Check sheet for the modelled part. Datum: model origin and axes. Units: mm. Coordinates: 2 decimals unless noted, no trailing zeros. Loops run counter-clockwise (first coordinate to the right, second up) from the corner with the lowest first, then second, coordinate; pieces in that order, holes last. Notation, with made-up numbers: M -32.5,21.5 L 19.5,21.5 A16 ccw 19.5,27.5 Z; hole C 24.5,71 d2. An arc over 180 degrees is marked long. Return JSON: item names as keys, results as strings.
from build123d import *

# Parameters (mm, degrees)
ESQUISSE1_R             = 40
ESQUISSE1_R_2           = 5.5
BOSS_EXTRU_1_DEPTH      = 10
BOSS_EXTRU_2_START      = -7
ESQUISSE2_R             = 40
BOSS_EXTRU_2_DEPTH      = 7
ESQUISSE3_R             = 15
BOSS_EXTRU_3_DEPTH      = 20
CONG_1_R                = 10
ESQUISSE4_R             = 4.875
ENL_V_MAT_EXTRU_1_DEPTH = 16


with BuildPart() as part:
    # Esquisse1 → Boss.-Extru.1 (new body)
    with BuildSketch(Plane.YZ):
        with Locations(Location((0, 0, 0), (0, 0, 270))):
            Circle(ESQUISSE1_R)
        with Locations(Location((0, 32, 0), (0, 0, 270))):
            Circle(ESQUISSE1_R_2, mode=Mode.SUBTRACT)
        with Locations(Location((12.245869836, 29.56414504, 0), (0, 0, 270))):
            Circle(ESQUISSE1_R_2, mode=Mode.SUBTRACT)
        with Locations(Location((22.627416998, 22.627416998, 0), (0, 0, 270))):
            Circle(ESQUISSE1_R_2, mode=Mode.SUBTRACT)
        with Locations(Location((29.56414504, 12.245869836, 0), (0, 0, 270))):
            Circle(ESQUISSE1_R_2, mode=Mode.SUBTRACT)
        with Locations(Location((32, 0, 0), (0, 0, 270))):
            Circle(ESQUISSE1_R_2, mode=Mode.SUBTRACT)
        with Locations(Location((29.56414504, -12.245869836, 0), (0, 0, 270))):
            Circle(ESQUISSE1_R_2, mode=Mode.SUBTRACT)
        with Locations(Location((22.627416998, -22.627416998, 0), (0, 0, 270))):
            Circle(ESQUISSE1_R_2, mode=Mode.SUBTRACT)
        with Locations(Location((12.245869836, -29.56414504, 0), (0, 0, 270))):
            Circle(ESQUISSE1_R_2, mode=Mode.SUBTRACT)
        with Locations(Location((0, -32, 0), (0, 0, 270))):
            Circle(ESQUISSE1_R_2, mode=Mode.SUBTRACT)
        with Locations(Location((-12.245869836, -29.56414504, 0), (0, 0, 270))):
            Circle(ESQUISSE1_R_2, mode=Mode.SUBTRACT)
        with Locations(Location((-22.627416998, -22.627416998, 0), (0, 0, 270))):
            Circle(ESQUISSE1_R_2, mode=Mode.SUBTRACT)
        with Locations(Location((-29.56414504, -12.245869836, 0), (0, 0, 270))):
            Circle(ESQUISSE1_R_2, mode=Mode.SUBTRACT)
        with Locations(Location((-32, 0, 0), (0, 0, 270))):
            Circle(ESQUISSE1_R_2, mode=Mode.SUBTRACT)
        with Locations(Location((-29.56414504, 12.245869836, 0), (0, 0, 270))):
            Circle(ESQUISSE1_R_2, mode=Mode.SUBTRACT)
        with Locations(Location((-22.627416998, 22.627416998, 0), (0, 0, 270))):
            Circle(ESQUISSE1_R_2, mode=Mode.SUBTRACT)
        with Locations(Location((-12.245869836, 29.56414504, 0), (0, 0, 270))):
            Circle(ESQUISSE1_R_2, mode=Mode.SUBTRACT)
        with Locations(Location((-11.429260712, 17.105097445, 0), (0, 0, 270))):
            Circle(ESQUISSE1_R_2, mode=Mode.SUBTRACT)
        with Locations(Location((4.013422643, 20.17683815, 0), (0, 0, 270))):
            Circle(ESQUISSE1_R_2, mode=Mode.SUBTRACT)
        with Locations(Location((17.105097445, 11.429260712, 0), (0, 0, 270))):
            Circle(ESQUISSE1_R_2, mode=Mode.SUBTRACT)
        with Locations(Location((20.17683815, -4.013422643, 0), (0, 0, 270))):
            Circle(ESQUISSE1_R_2, mode=Mode.SUBTRACT)
        with Locations(Location((11.429260712, -17.105097445, 0), (0, 0, 270))):
            Circle(ESQUISSE1_R_2, mode=Mode.SUBTRACT)
        with Locations(Location((-4.013422643, -20.17683815, 0), (0, 0, 270))):
            Circle(ESQUISSE1_R_2, mode=Mode.SUBTRACT)
        with Locations(Location((-17.105097445, -11.429260712, 0), (0, 0, 270))):
            Circle(ESQUISSE1_R_2, mode=Mode.SUBTRACT)
        with Locations(Location((-20.17683815, 4.013422643, 0), (0, 0, 270))):
            Circle(ESQUISSE1_R_2, mode=Mode.SUBTRACT)
        with Locations(Location((5.527683242, 8.272762594, 0), (0, 0, 270))):
            Circle(ESQUISSE1_R_2, mode=Mode.SUBTRACT)
        with Locations(Location((8.272762594, -5.527683242, 0), (0, 0, 270))):
            Circle(ESQUISSE1_R_2, mode=Mode.SUBTRACT)
        with Locations(Location((-5.527683242, -8.272762594, 0), (0, 0, 270))):
            Circle(ESQUISSE1_R_2, mode=Mode.SUBTRACT)
        with Locations(Location((-8.272762594, 5.527683242, 0), (0, 0, 270))):
            Circle(ESQUISSE1_R_2, mode=Mode.SUBTRACT)
    extrude(amount=BOSS_EXTRU_1_DEPTH)

    # Esquisse2 → Boss.-Extru.2 (add)
    with BuildSketch(Plane.YZ.offset(10).offset(BOSS_EXTRU_2_START)):
        with Locations(Location((0, 0, 0), (0, 0, 270))):
            Circle(ESQUISSE2_R)
    extrude(amount=BOSS_EXTRU_2_DEPTH)

    # Esquisse3 → Boss.-Extru.3 (add)
    with BuildSketch(Plane.YZ.offset(10)):
        with Locations(Location((0, 0, 0), (0, 0, 270))):
            Circle(ESQUISSE3_R)
    extrude(amount=BOSS_EXTRU_3_DEPTH)

    # Congé1
    cong_1_edges = [part.edges().sort_by_distance(p)[0] for p in [
        (10, 0, 15),
    ]]
    fillet(cong_1_edges, radius=CONG_1_R)

    # Esquisse4 → Enlèv. mat.-Extru.1 (cut)
    with BuildSketch(Plane.YZ.offset(30)):
        with Locations(Location((0, 0, 0), (0, 0, 270))):
            Circle(ESQUISSE4_R)
    extrude(amount=-ENL_V_MAT_EXTRU_1_DEPTH, mode=Mode.SUBTRACT)


solid = part.part
1) Draft check along Y on faces 1 (the face through (1.48, 12.49, 35.06)), 2 (the face through (0, 1, 1)). Enter one of: +Y half, -Y half, draft (parallel to the pull), parting line (faces both ways), or undercut.
Answers:
{"face 1": "undercut", "face 2": "draft"}
2) Section check B-B on y = -32. Record the cut outline in (x, z).
Answers:
{"outline": "M 0,-24 L 10,-24 L 10,24 L 0,24 L 0,17.18 L 3,17.18 L 3,7.31 L 0,7.31 L 0,5.5 L 3,5.5 L 3,-5.5 L 0,-5.5 L 0,-7.31 L 3,-7.31 L 3,-17.18 L 0,-17.18 Z"}
3) Section check A-A on x = 26.25. Record the cut outline in (y, z) (3 decimals).
Answers:
{"outline": "C 0,0 d30; hole C 0,0 d9.75"}
4) Section check D-D on x = 18.5. Record the cut outline in (y, z) (3 decimals), then the cut area to 3 significant figures.
Answers:
{"outline": "C 0,0 d30.226; hole C 0,0 d9.75", "area": "643 mm²"}
5) Scan lines: line 1 along Z through (x, y) = (1.75, 18.5); line 2 along X through (y, z) = (-6.5, -8.5); line 3 along X through (y, z) = (13.5, -36). Record each from-to range of solid material in increasing order. Write a range as [from, to].
Answers:
{"line 1": "[-35.46, -26.26], [-18.99, -9.25], [1.22, 6.11], [16.75, 18.99], [26.26, 35.46]", "line 2": "[3, 30]", "line 3": "[0, 10]"}
6) Section check C-C on x = 8.5. Record the cut outline in (y, z).
Answers:
{"outline": "C 0,0 d80"}
7) Go/stop test with flat-tipped pins: pin 1 Ø1.5 at (y, z) = (9.5, 32) entering from +X; pin 2 Ø5 at (x, z) = (10, -4.5) entering from +Y; pin 3 Ø3 at (x, z) = (18.5, -18.5) entering from +Y; pin 4 Ø17.5 at (y, z) = (-12.25, -29.56) entering from +X. Record where each tip stops, or that it passes through.
Answers:
{"pin 1": "x = 10", "pin 2": "y = 39.95", "pin 3": "through", "pin 4": "x = 10.15"}
